Work out the finished part from the listing and answer in its coordinate system (mm). A direction names the side the tool comes from. Give positions to 0.01 mm unless a question says otherwise; leave off trailing zeros. Write each loop counter-clockwise with the first axis right and the second up, starting at its lowest first coordinate (ties: lowest second). Pieces come first, ordered by that corner, then holes. Notation, with made-up numbers: (44, 58) -> (61, 58) arc R17 ccw to (61, 73) -> close; hole circle Ø2 at (75.5, 76). An arc over 180 degrees is marked (long way). Use a Markdown table: item, result. Add a question column.
Q1. Section C-C, the plane x = 0 is taken. Give the vertices of the cut face in (y, z), plus the area to 3 significant figures.
Q2. For a pull along Z with two mould halves and no side action, classify faces 4 (the face through (2.75, 2.5, 12.4)), 5 (the face through (-3, 0, 6)), 6 (the face through (0, 3, -8.89)) as pulls with the +Z half, pulls with the -Z half, needs draft (parallel to the pull), parting line crosses it, or undercut.
Q3. Section A-A, the plane z = 0 is taken. Give the vertices of the cut face in (x, y), plus the area to 3 significant figures.
Q4. Each of these flat-tipped pins is pushed along its axis until it touches: pin 1 Ø1.1 at (y, z) = (4, -4.5) entering from -X; pin 2 Ø3 at (y, z) = (0, -5) entering from +X; pin 3 Ø4 at (x, z) = (-2, 8.5) entering from +Y; pin 4 Ø1 at (x, y) = (8.5, -6) entering from +Z. Where does it stop, or does it pass through?
Q5. Section D-D, the plane y = -14 is taken. Give the vertices of the cut face in (x, z).
Q6. For faces 1 (the face through (-1.38, -18.78, 6.2)), 2 (the face through (8.89, 3, 0)), 3 (the face through (-0.9, 5.08, -9.3)), determine the directions among +Z, -Z, +X, -X, +Y, -Y from which every point of the face is accessible in a straight line to the end or side of a thin tool.
Q7. Consider line 1 (Y direction, x = 9, z = -5.25); line 2 (Y direction, x = -2.5, z = -6); line 3 (Z direction, x = 2.75, y = 1.5). Determine where each line is inside the solid, lowest interval first.
Q8. Section B-B, the plane y = 2 is taken. Give the vertices of the cut face in (x, z).
Autodesk Inventor part; units mm, degrees
ref_plane "YZ Plane" through (0, 0, 0) normal (1, 0, 0) x (0, 1, 0)
ref_plane "XZ Plane" through (0, 0, 0) normal (0, 1, 0) x (-1, 0, 0)
ref_plane "XY Plane" through (0, 0, 0) normal (0, 0, 1) x (1, 0, 0)
sketch "Sketch1" plane through (0, 0, 0) normal (0, 1, 0) x (-1, 0, 0)
  circle A0 centre (0, 0) radius 12.7
  dimension "d0" = 25.4
extrude "Extrusion1" add sketch "Sketch1" along normal blind 5.08
sketch "Sketch2" plane through (0, 5.08, 0) normal (0, 1, 0) x (1, 0, 0)
  line L0 (-8.89, -8.89) -> (8.89, -8.89)
  line L1 (8.89, -8.89) -> (8.89, 8.89)
  line L2 (8.89, 8.89) -> (-8.89, 8.89)
  line L3 (-8.89, 8.89) -> (-8.89, -8.89)
  point P0 (0, 0)
extrude "Extrusion2" cut sketch "Sketch2" against normal blind 3.81
sketch "Sketch3" plane through (0, 0, 0) normal (0, -1, 0) x (1, 0, 0)
  circle A0 centre (0, 0) radius 6.35
  dimension "d9" = 12.7
extrude "Extrusion3" add sketch "Sketch3" along normal blind 38.1
thread "Thread1"
properties part number "Bolt"
Result set:
| question | item | result |
|---|---|---|
| 1 | outline | (-38.1, -6.35) -> (0, -6.35) -> (0, -12.7) -> (5.08, -12.7) -> (5.08, -8.89) -> (1.27, -8.89) -> (1.27, 8.89) -> (5.08, 8.89) -> (5.08, 12.7) -> (0, 12.7) -> (0, 6.35) -> (-38.1, 6.35) -> close |
| 1 | area | 545 mm2 |
| 2 | face 4 | parting line crosses it |
| 2 | face 5 | needs draft |
| 2 | face 6 | undercut |
| 3 | outline | (-12.7, 0) -> (-6.35, 0) -> (-6.35, -38.1) -> (6.35, -38.1) -> (6.35, 0) -> (12.7, 0) -> (12.7, 5.08) -> (8.89, 5.08) -> (8.89, 1.27) -> (-8.89, 1.27) -> (-8.89, 5.08) -> (-12.7, 5.08) -> close |
| 3 | area | 545 mm2 |
| 4 | pin 1 | stops at x = -12.07 |
| 4 | pin 2 | stops at x = 12.21 |
| 4 | pin 3 | stops at y = 5.08 |
| 4 | pin 4 | passes through |
| 5 | outline | circle Ø12.7 at (0, 0) |
| 6 | face 1 | -Y |
| 6 | face 2 | +Y |
| 6 | face 3 | +Z, -Z, +X, -X, +Y |
| 7 | line 1 | y = 0 to 5.08 |
| 7 | line 2 | y = 0 to 1.27 |
| 7 | line 3 | z = -12.4 to -8.89, 8.89 to 12.4 |
| 8 | outline | circle Ø25.4 at (0, 0); hole (-8.89, -8.89) -> (8.89, -8.89) -> (8.89, 8.89) -> (-8.89, 8.89) -> close |
